Could you check a few things on this model? Use its own coordinates, in mm. A direction names the side the tool comes from. Give positions to 0.01 mm unless a question says otherwise; leave off trailing zeros. Loops run counter-clockwise (first coordinate to the right, second up) from the corner with the lowest first, then second, coordinate; pieces in that order, holes last. Notation, with made-up numbers: M -23.75,36.5 L -15.75,36.5 A26 ccw -15.75,74.5 Z; hole C -19.5,-26.75 d6. An arc over 180 degrees is marked long. Answer in a Markdown table with one row per item. Add a question column.
```python
from build123d import *

# Parameters (mm, degrees)
BOSS_EXTRUDE1_DEPTH = 20
SKETCH3_W           = 35
SKETCH3_H           = 18.5
CUT_EXTRUDE2_DEPTH  = 44.406131606
CUT_EXTRUDE1_DEPTH  = 17
SKETCH5_R           = 1.75
CUT_EXTRUDE4_DEPTH  = 44.406131606
SKETCH6_R           = 3.75
CUT_EXTRUDE5_DEPTH  = 7
CHAMFER1_SIZE       = 2
FILLET1_R           = 5
BOSS_EXTRUDE5_DEPTH = 2
CHAMFER2_SIZE       = 2
FILLET2_R           = 2
SKETCH8_W           = 2
SKETCH8_H           = 17.504208533
CUT_EXTRUDE6_DEPTH  = 3


# Some blends are built 0.0001 mm under size
with BuildPart() as part:
    # Sketch1 → Boss-Extrude1 (new body)
    with BuildSketch(Plane.XY):
        with BuildLine():
            Line((-22.5, 0), (22.5, 0))
            ThreePointArc((22.5, 0), (26.035533906, -1.464466094), (27.5, -5))
            Line((27.5, -5), (27.5, -13.096343094))
            ThreePointArc((27.5, -13.096343094), (29.304354621, -15.847784921), (32.546954751, -15.289508899))
            Line((32.546954751, -15.289508899), (35, -13))
            Line((35, -13), (35, -4))
            Line((35, -4), (27.5, 10))
            Line((27.5, 10), (-27.5, 10))
            Line((-27.5, 10), (-35, -4))
            Line((-35, -4), (-35, -13))
            Line((-35, -13), (-32.546954751, -15.289508899))
            ThreePointArc((-32.546954751, -15.289508899), (-29.304354621, -15.847784921), (-27.5, -13.096343094))
            Line((-27.5, -13.096343094), (-27.5, -5))
            ThreePointArc((-27.5, -5), (-26.035533906, -1.464466094), (-22.5, 0))
        make_face()
    extrude(amount=BOSS_EXTRUDE1_DEPTH)

    # Sketch3 → Cut-Extrude2 (cut, through all)
    with BuildSketch(Plane.XZ):
        with Locations((0, 10.75)):
            Rectangle(SKETCH3_W, SKETCH3_H)
    extrude(amount=-CUT_EXTRUDE2_DEPTH, mode=Mode.SUBTRACT)

    # Sketch2 → Cut-Extrude1 (cut)
    with BuildSketch(Plane.XY.offset(20)):
        with BuildLine():
            Line((-27.5, -13.096343094), (-30.529524623, -13.096343094))
            Line((-30.529524623, -13.096343094), (-31, -13.096343094))
            ThreePointArc((-31, -13.096343094), (-32.414213562, -12.510556657), (-33, -11.096343094))
            Line((-33, -11.096343094), (-33, 8.594773791))
            Line((-33, 8.594773791), (-29.5, 8.594773791))
            Line((-29.5, 8.594773791), (-29.5, -7.096343094))
            Line((-29.5, -7.096343094), (-27.5, -7.096343094))
            Line((-27.5, -7.096343094), (-27.5, -13.096343094))
        make_face()
    cut_extrude1 = extrude(amount=-CUT_EXTRUDE1_DEPTH, mode=Mode.SUBTRACT)

    # Mirror1: Cut-Extrude1 across plane
    add(cut_extrude1.mirror(Plane(origin=(0, 0, 0), x_dir=(0, 0, 1), z_dir=(1, 0, 0))), mode=Mode.SUBTRACT)

    # Sketch5 → Cut-Extrude4 (cut, through all)
    with BuildSketch(Plane.XY.offset(20)):
        with Locations((-23, 5)):
            Circle(SKETCH5_R)
        with Locations((23, 5)):
            Circle(SKETCH5_R)
    extrude(amount=-CUT_EXTRUDE4_DEPTH, mode=Mode.SUBTRACT)

    # Sketch6 → Cut-Extrude5 (cut)
    with BuildSketch(Plane.XY.offset(20)):
        with Locations((-23, 5)):
            Circle(SKETCH6_R)
        with Locations((23, 5)):
            Circle(SKETCH6_R)
    extrude(amount=-CUT_EXTRUDE5_DEPTH, mode=Mode.SUBTRACT)

    # Chamfer1
    # the kernel refuses this chamfer: 2 mm, written as the material it takes off along each edge
    with BuildSketch(Plane(origin=(17.5, 0, 1.5), x_dir=(0, -0.027495876610586365, -0.9996219169112968), z_dir=(-1, 0, 0))) as chamfer1_piece_1:
        Polygon((CHAMFER1_SIZE * 0.999621916911, -CHAMFER1_SIZE * 0.0274958766106), (-CHAMFER1_SIZE * 0.0274958766106, -CHAMFER1_SIZE * 0.999621916911), (0, 0), align=None)
    extrude(amount=35, mode=Mode.SUBTRACT)

    # Fillet1
    fillet1_edges = [part.edges().sort_by_distance(p)[0] for p in [
        (-17.5, 6, 1.5),
        (17.5, 6, 1.5),
    ]]
    fillet(fillet1_edges, radius=FILLET1_R)

    # Sketch7 → Boss-Extrude5 (add, symmetric)
    with BuildSketch(Plane(origin=(-27.5, 0, 0), x_dir=(0, 0, -1), z_dir=(1, 0, 0))):
        with BuildLine():
            Line((0, -10.096343094), (0, 0))
            Line((0, 0), (-10.6, 0))
            Line((-10.6, 0), (-10.6, -7.496343094))
            Line((-10.6, -7.496343094), (-5.6, -7.496343094))
            ThreePointArc((-5.6, -7.496343094), (-3, -10.096343094), (-5.6, -12.696343094))
            Line((-5.6, -12.696343094), (-10.6, -12.696343094))
            Line((-10.6, -12.696343094), (-10.6, -15.696343094))
            Line((-10.6, -15.696343094), (-5.6, -15.696343094))
            ThreePointArc((-5.6, -15.696343094), (-1.640202025, -14.056141069), (0, -10.096343094))
        make_face()
    boss_extrude5 = extrude(amount=BOSS_EXTRUDE5_DEPTH, both=True)

    # Mirror4: Boss-Extrude5 across plane
    add(boss_extrude5.mirror(Plane(origin=(0, 0, 0), x_dir=(0, 0, 1), z_dir=(1, 0, 0))))

    # Chamfer2
    chamfer2_edges = [part.edges().sort_by_distance(p)[0] for p in [
        (25.5, -14.196343094, 10.6),
        (25.5, -4.248171547, 10.6),
        (-25.5, -4.248171547, 10.6),
        (-25.5, -14.196343094, 10.6),
    ]]
    chamfer(chamfer2_edges, length=CHAMFER2_SIZE - 0.0001)  # a hair under: the kernel refuses the full size

    # Fillet2
    fillet2_edges = [part.edges().sort_by_distance(p)[0] for p in [
        (25.5, -5.548171547, 0),
        (25.5, -14.056141069, 1.640202025),
        (-25.5, -5.548171547, 0),
        (-25.5, -14.056141069, 1.640202025),
        (25.5, -15.696343094, 7.10005),
        (-25.5, -15.696343094, 7.10005),
    ]]
    fillet(fillet2_edges, radius=FILLET2_R - 0.0001)  # a hair under: the kernel refuses the full size

    # Sketch8 → Cut-Extrude6 (cut)
    with BuildSketch(Plane(origin=(-25.530227948, 13.67690783, 0), x_dir=(0, 0, 1), z_dir=(-0.8814799700287818, 0.4722214125154193, 0))):
        with Locations((4, -6.39655042)):
            Rectangle(SKETCH8_W, SKETCH8_H)
    cut_extrude6 = extrude(amount=-CUT_EXTRUDE6_DEPTH, mode=Mode.SUBTRACT)

    # Mirror5: Cut-Extrude6 across plane
    add(cut_extrude6.mirror(Plane(origin=(0, 0, 0), x_dir=(0, 0, 1), z_dir=(1, 0, 0))), mode=Mode.SUBTRACT)


solid = part.part
```
Item 1: If we mould it in two halves opening along X, with no side actions, what happens to faces 1 (the face through (-26.1, -5.48, 0.57)), 2 (the face through (-28.486, 8.159, 12.395)), 3 (the face through (27, -12.696, 8)), 4 (the face through (28.514, 8.107, 12.395))? For each: +X half, -X half, draft (parallel to the pull), parting line (faces both ways), or undercut.
Item 2: Suppose I cut it at B-B (y = 5). Give the number of separate pieces and of enclosed holes in the cut face, then the cut area to 3 significant figures.
Item 3: For faces 5 (the face through (-25.5, -6, 5)), 6 (the face through (-27, -7.496, 8)), 7 (the face through (-29.5, 0, 12)), which set-ups out of +Z, -Z, +X, -X, +Y, -Y let a thin tool reach every point of the face, with its end or its side?
Item 4: I need wall thicknesses on L1, parallel to X at y = -11, z = 7.75; L2, parallel to X at y = -6.75, z = 3.25; L3, parallel to X at y = 5.5, z = 15. Which ranges of each line are inside material? Lowest first, please.
Item 5: Suppose I cut it at A-A (x = 5.5). List the corners of the cut face in (y, z) for me.
Item 6: For P1, Ø1.7, axis at x = -28, z = 8.5, coming from the -Y side; P2, Ø4, axis at x = 22.5, y = 4, coming from the +Z side; P3, Ø3, axis at y = 3, z = 11.5, coming from the -X side, each with a flat end and sliding along its axis, tell me the tip position at first contact or that it passes through.
Values found:
| question | item | result |
|---|---|---|
| 1 | face 1 | undercut |
| 1 | face 2 | -X half |
| 1 | face 3 | undercut |
| 1 | face 4 | +X half |
| 2 | separate pieces | 3 |
| 2 | enclosed holes | 0 |
| 2 | area | 340 mm² |
| 3 | face 5 | +Z, -Z, -Y |
| 3 | face 6 | +Z |
| 3 | face 7 | +Z, +Y |
| 4 | L1 | -35 to -33, 33 to 35 |
| 4 | L2 | -35 to -33, -29.5 to -25.5, 25.5 to 29.5, 33 to 35 |
| 4 | L3 | -29.5 to -26.72, -19.28 to -17.5, 17.5 to 19.28, 26.72 to 29.5 |
| 5 | outline | M 0.5,0 L 10,0 L 10,1.5 L 2,1.5 Z |
| 6 | P1 | y = -15.7 |
| 6 | P2 | z = 13 |
| 6 | P3 | x = -29.5 |
